Here's how the part is built. I have some questions about the finished solid (model axes, mm). Face numbers are marked on the shaded views. A direction names the side the tool comes from. Round coordinates to 2 decimals unless told otherwise and drop trailing zeros. Write each loop counter-clockwise with the first axis right and the second up, starting at its lowest first coordinate (ties: lowest second). Pieces come first, ordered by that corner, then holes. Notation, with made-up numbers: (13, 18) -> (24, 18) arc R20 ccw to (24, 55) -> close; hole circle Ø7 at (2, 86). An arc over 180 degrees is marked (long way). Put each result on its own line as item: value. Start each with the question number.
1) If I drill on line 1 along X through (y, z) = (18.5, 1.5); line 2 along Y through (x, z) = (-39.8, -20); line 3 along Z through (x, y) = (37, 14.5), over which ranges is the centre line in solid material (lowest first)? Write a range as [from, to].
2) Which directions (+Z, -Z, +X, -X, +Y, -Y) give clear straight access to the entire face, cutting with the end or side of a thin tool? Please do the marked faces 5 and 6.
3) I want a section at C-C, the plane y = 0. List the corners of the cut face in (x, z) for me.
4) I want a section at B-B, the plane y = -4. List the corners of the cut face in (x, z) for me, then the cut area to 3 significant figures.
5) I want a section at A-A, the plane z = -3. List the corners of the cut face in (x, y) for me, then the cut area to 3 significant figures.
6) Will this pin go through, and if not, where does the flat tip stop? P1, Ø12, axis at x = 6, y = -10.5, coming from the -Z side.
7) We'd pull the mould along X, two halves only. Please class the marked faces 1, 2, 3 and 4: released by +X, released by -X, zero draft, split by the parting line, or undercut.
8) I want a section at D-D, the plane z = -20. List the corners of the cut face in (x, y) for me.
Autodesk Inventor part; units mm, degrees
ref_plane "YZ Plane" through (0, 0, 0) normal (1, 0, 0) x (0, 1, 0)
ref_plane "XZ Plane" through (0, 0, 0) normal (0, 1, 0) x (-1, 0, 0)
ref_plane "РабПлоскость1" through (0, 0, 24) normal (0, 0, 1) x (1, 0, 0)
sketch "Эскиз1" plane through (0, 0, 24) normal (0, 0, 1) x (1, 0, 0)
  line L0 (-40, 20) -> (40, 20)
  line L1 (40, 20) -> (40, -20)
  line L2 (40, -20) -> (-40, -20)
  line L3 (-40, -20) -> (-40, 20)
  line L4 (-40, 20) -> (40, -20) construction
  line L5 (40, 20) -> (-40, -20) construction
  point P0 (0, 0)
  dimension "d1" = 80
  dimension "d2" = 40
extrude "Пластина1" add sketch "Эскиз1" against normal blind 0.5
sketch "Эскиз2" plane through (-39.5, 20, 24) normal (-1, 0, 0) x (0, -1, 0)
  line L0 (40, 0) -> (0, 0)
  line L1 (0, 0) -> (0, -47.5)
  line L2 (0, -47.5) -> (40, -47.5)
  line L3 (40, -47.5) -> (40, 0)
edge flange "Фланец1" height 47.5 angle 90 thickness 0.5 bend radius 0.5 thickness toward (-1, 0, 0) relief tear relief width 0.5 relief depth 0.25 corner gap 0.5 corner form 0 edges at (-40, 0, 23.5) (40, 0, 23.5) wall of the first edge with corners at (-39.5, -20, 24) (-39.5, 20, 24) (-39.5, 20, -23.5) (-39.5, -20, -23.5)
bend "Сгиб1"
corner "УглСтык1"
sketch "Эскиз3" plane through (0, 0, 24) normal (0, 0, 1) x (1, 0, 0)
  line L0 (19.5, -10.85) -> (14, -10.85)
  line L1 (14, -10.85) -> (14, 10.85)
  line L2 (14, 10.85) -> (19.5, 10.85)
  line L3 (19.5, 10.85) -> (19.5, -10.85)
  line L4 (19.5, -10.85) -> (14, 10.85) construction
  line L5 (14, -10.85) -> (19.5, 10.85) construction
  line L6 (14.5, -10.5) -> (18.5, -10.5)
  line L7 (14.5, -10.5) -> (14.5, -9)
  line L8 (18.5, -10.5) -> (18.5, -9)
  line L9 (18.5, -9) -> (14.5, -9)
  line L10 (14.5, 9) -> (18.5, 9)
  line L11 (14.5, 9) -> (14.5, 10.5)
  line L12 (14.5, 10.5) -> (18.5, 10.5)
  line L13 (18.5, 9) -> (18.5, 10.5)
  line L14 (13.98, 11.925) -> (17.88, 11.925)
  line L15 (18.38, 10.5) -> (18.38, 11.925)
  line L16 (17.88, -11.925) -> (13.98, -11.925)
  line L17 (18.38, -11.925) -> (18.38, -10.5)
  line L18 (19.5, 9) -> (19.5, -9)
  line L19 (19.5, -10.5) -> (19.5, -9)
  line L20 (19.5, -10.5) -> (18.5, -10.5)
  line L21 (19.5, 9) -> (18.5, 9)
  line L22 (34.5, -2.5) -> (34.5, 2.5)
  line L23 (34.5, 0) -> (19.5, 0)
  point P0 (0, 0)
  point P1 (16.75, 0)
  point P2 (14, 0)
  dimension "d14" = 5.5
  dimension "d15" = 21.7
  dimension "d19" = 15
fillet "УглСкругление1" radius 0.5 4 edges at (-39.75, 20, -23.5) (-39.75, -20, -23.5) (39.75, 20, -23.5) (39.75, -20, -23.5)
extrude "Вырез1" cut sketch "Эскиз3" against normal blind 0.5
sketch "Эскиз4" plane through (-40, -20, 23) normal (-1, 0, 0) x (0, 0, 1)
  circle A0 centre (-43, 20) radius 1.5
  circle A1 centre (-43, 20) radius 1.1
  point P0 (-23, 20)
  dimension "d20" = 2.2
extrude "Вырез2" cut sketch "Эскиз4" against normal blind 80 contours A1
sketch "Эскиз5" plane through (0, 0, 24) normal (0, 0, 1) x (1, 0, 0)
  line L0 (19.5, 10.85) -> (19.5, -10.85)
  line L1 (19.5, -10.85) -> (14, -10.85)
  line L2 (14, -10.85) -> (14, 10.85)
  line L3 (14, 10.85) -> (19.5, 10.85)
  line L4 (39, -20) -> (39, 20)
  line L5 (-39, 20) -> (39, 20)
  line L6 (-39, 20) -> (-39, -20)
  line L7 (39, -20) -> (-39, -20)
  line L8 (-40, -20) -> (-40, 20)
  line L9 (-40, -20) -> (-39, -20)
  line L10 (-39, 20) -> (-40, 20)
  line L11 (39, -20) -> (40, -20)
  line L12 (40, 20) -> (40, -20)
  line L13 (40, 20) -> (39, 20)
  point P0 (0, 0)
sketch "Эскиз6" plane through (-40, -20, 23) normal (-1, 0, 0) x (0, 0, 1)
  circle A0 centre (-43, 20) radius 1.1
  arc A1 (-46, 40) -> (-46.5, 39.5) centre (-46, 39.5) ccw
  line L0 (-46.5, 0.5) -> (-46.5, 39.5)
  arc A2 (-46.5, 0.5) -> (-46, 0) centre (-46, 0.5) ccw
  line L1 (0, 0) -> (-46, 0)
  line L2 (0, 0) -> (0, 40)
  line L3 (-46, 40) -> (0, 40)
  point P0 (-23, 20)
equation "\"d17\" = Толщина"
equation "\"d3\" = Толщина"
equation "\"d4\" = Ширина_просечки"
equation "\"d5\" = Глубина_просечки"
equation "\"d6\" = Мин_остаток"
equation "\"d7\" = Радиус_перехода"
equation "\"d10\" = Радиус_гибки"
equation "\"d11\" = Размер_просечки"
equation "\"d12\" = Размер_зазора"
equation "\"d13\" = Радиус_Якоби"
equation "\"Радиус_гибки\" = Толщина"
equation "\"Ширина_просечки\" = Толщина"
equation "\"Глубина_просечки\" = 0.5 * Толщина"
equation "\"Размер_просечки\" = 4 * Толщина"
equation "\"Мин_остаток\" = 2 * Толщина"
equation "\"Радиус_перехода\" = Радиус_гибки"
equation "\"Радиус_Якоби\" = Радиус_гибки"
equation "\"Размер_зазора\" = Толщина"
properties part number "metal_cap"
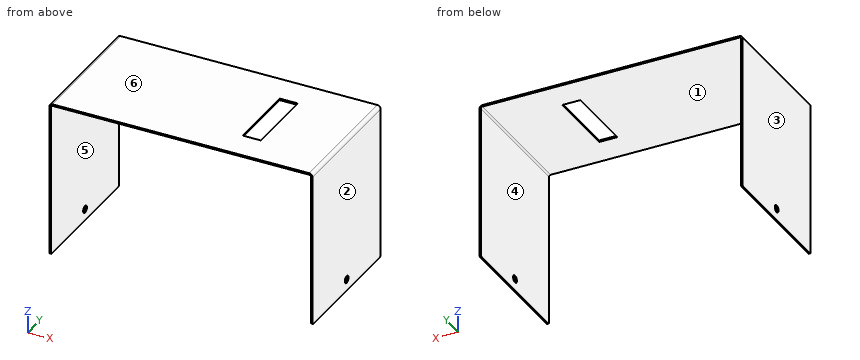
Findings:
1. line 1: x = [-40, -39.5], [39.5, 40]
1. line 2: y = [-20, -1.1], [1.1, 20]
1. line 3: z = [23.5, 24]
2. face 5: -Z, +Y, -Y
2. face 6: +Z, +X, -X, +Y, -Y
3. outline: (-40, -23.5) -> (-39.5, -23.5) -> (-39.5, -21.1) -> (-40, -21.1) -> close; (-40, -18.9) -> (-39.5, -18.9) -> (-39.5, 23) arc R0.5 cw to (-39, 23.5) -> (14, 23.5) -> (14, 24) -> (-39, 24) arc R1 ccw to (-40, 23) -> close; (19.5, 23.5) -> (39, 23.5) arc R0.5 cw to (39.5, 23) -> (39.5, -18.9) -> (40, -18.9) -> (40, 23) arc R1 ccw to (39, 24) -> (19.5, 24) -> close; (39.5, -23.5) -> (40, -23.5) -> (40, -21.1) -> (39.5, -21.1) -> close
4. outline: (-40, -23.5) -> (-39.5, -23.5) -> (-39.5, 23) arc R0.5 cw to (-39, 23.5) -> (14, 23.5) -> (14, 24) -> (-39, 24) arc R1 ccw to (-40, 23) -> close; (19.5, 23.5) -> (39, 23.5) arc R0.5 cw to (39.5, 23) -> (39.5, -23.5) -> (40, -23.5) -> (40, 23) arc R1 ccw to (39, 24) -> (19.5, 24) -> close
4. area: 83.9 mm2
5. outline: (-40, -20) -> (-39.5, -20) -> (-39.5, 20) -> (-40, 20) -> close; (39.5, -20) -> (40, -20) -> (40, 20) -> (39.5, 20) -> close
5. area: 40.0 mm2
6. P1: stops at z = 23.5
7. face 1: undercut
7. face 2: released by +X
7. face 3: released by -X
7. face 4: undercut
8. outline: (-40, -20) -> (-39.5, -20) -> (-39.5, -1.1) -> (-40, -1.1) -> close; (-40, 1.1) -> (-39.5, 1.1) -> (-39.5, 20) -> (-40, 20) -> close; (39.5, -20) -> (40, -20) -> (40, -1.1) -> (39.5, -1.1) -> close; (39.5, 1.1) -> (40, 1.1) -> (40, 20) -> (39.5, 20) -> close
